Check sheet for the modelled part. Datum: model origin and axes. Units: mm. Face numbers are marked on the shaded views. A direction names the side the tool comes from. Round coordinates to 2 decimals unless told otherwise and drop trailing zeros. Write each loop counter-clockwise with the first axis right and the second up, starting at its lowest first coordinate (ties: lowest second). Pieces come first, ordered by that corner, then holes. Notation, with made-up numbers: M 73,-34 L 113,-34 A19 ccw 113,-1 Z; hole C 80.5,38 d1. An arc over 180 degrees is marked long. Answer in a Markdown table with one row per item.
```python
from build123d import *

# Parameters (mm, degrees)
SKETCH1_W           = 10
SKETCH1_H           = 80
BOSS_EXTRUDE1_DEPTH = 20
FILLET1_R           = 5
SKETCH3_R           = 3.99
BOSS_EXTRUDE2_DEPTH = 8.5
SKETCH4_R           = 5.65
BOSS_EXTRUDE3_DEPTH = 1.5
SKETCH2_R           = 5.65
BOSS_EXTRUDE4_DEPTH = 3
SKETCH6_R           = 3.99
BOSS_EXTRUDE5_DEPTH = 7.5
BOSS_EXTRUDE6_START = 3
SKETCH7_R           = 5.65
BOSS_EXTRUDE6_DEPTH = 3
BOSS_EXTRUDE7_START = 7.5
SKETCH9_R           = 3.99
BOSS_EXTRUDE7_DEPTH = 7.5


with BuildPart() as part:
    # Sketch1 → Boss-Extrude1 (new body)
    with BuildSketch(Plane(origin=(0, 0, 0), x_dir=(1, 0, 0), z_dir=(0, 1, 0))):
        with Locations((5, 40)):
            Rectangle(SKETCH1_W, SKETCH1_H)
    extrude(amount=BOSS_EXTRUDE1_DEPTH)

    # Fillet1
    fillet1_edges = [part.edges().sort_by_distance(p)[0] for p in [
        (5, 0, 0),
        (5, 20, 0),
    ]]
    fillet(fillet1_edges, radius=FILLET1_R)

    # Sketch3 → Boss-Extrude2 (add)
    with BuildSketch(Plane(origin=(0, 0, -80), x_dir=(-1, 0, 0), z_dir=(0, 0, -1))):
        with Locations(Location((-5, 10, 0), (0, 0, 180))):
            Circle(SKETCH3_R)
    extrude(amount=BOSS_EXTRUDE2_DEPTH)

    # Sketch4 → Boss-Extrude3 (add)
    with BuildSketch(Plane(origin=(0, 0, -80), x_dir=(-1, 0, 0), z_dir=(0, 0, -1))):
        with Locations(Location((-5, 10, 0), (0, 0, 207.753923356))):
            Circle(SKETCH4_R)
    extrude(amount=BOSS_EXTRUDE3_DEPTH)

    # Sketch2 → Boss-Extrude4 (add)
    with BuildSketch(Plane(origin=(10, 0, 0), x_dir=(0, 0, -1), z_dir=(1, 0, 0))):
        with Locations(Location((10, 10, 0), (0, 0, 180))):
            Circle(SKETCH2_R)
    extrude(amount=BOSS_EXTRUDE4_DEPTH)

    # Sketch6 → Boss-Extrude5 (add)
    with BuildSketch(Plane(origin=(13, 0, 0), x_dir=(0, 0, -1), z_dir=(1, 0, 0))):
        with Locations((10, 10)):
            Circle(SKETCH6_R)
    extrude(amount=BOSS_EXTRUDE5_DEPTH)

    # Sketch7 → Boss-Extrude6 (add)
    with BuildSketch(Plane.ZY.offset(BOSS_EXTRUDE6_START)):
        with Locations((-10, 10)):
            Circle(SKETCH7_R)
    extrude(amount=-BOSS_EXTRUDE6_DEPTH)

    # Sketch9 → Boss-Extrude7 (add)
    with BuildSketch(Plane.ZY.offset(3).offset(BOSS_EXTRUDE7_START)):
        with Locations(Location((-10, 10, 0), (0, 0, 180))):
            Circle(SKETCH9_R)
    extrude(amount=-BOSS_EXTRUDE7_DEPTH)


solid = part.part
```
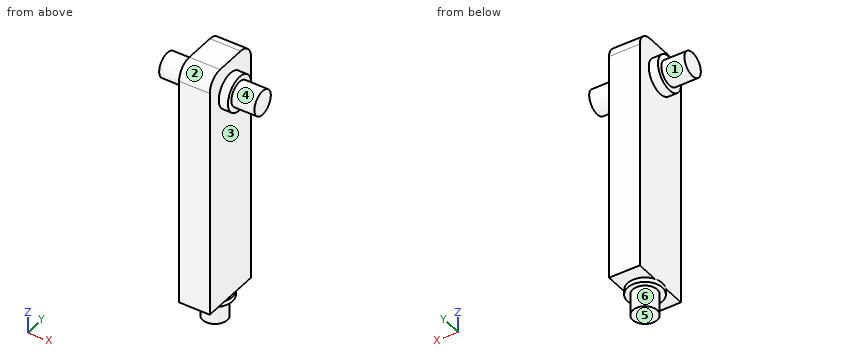
1. Access from +Z, -Z, +X, -X, +Y, -Y to the whole of each face (thin tool, end or side, straight path). Record for the marked faces 4, 5 and 6.
Found:
| item | result |
|---|---|
| face 4 | +X |
| face 5 | -Z, +X, -X, +Y, -Y |
| face 6 | -Z |
2. Section check A-A, the plane y = 10. Record the cut outline in (x, z).
Found:
| item | result |
|---|---|
| outline | M -10.5,-13.99 L -3,-13.99 L -3,-15.65 L 0,-15.65 L 0,-80 L -0.65,-80 L -0.65,-81.5 L 1.01,-81.5 L 1.01,-88.5 L 8.99,-88.5 L 8.99,-81.5 L 10.65,-81.5 L 10.65,-80 L 10,-80 L 10,-15.65 L 13,-15.65 L 13,-13.99 L 20.5,-13.99 L 20.5,-6.01 L 13,-6.01 L 13,-4.35 L 10,-4.35 L 10,0 L 0,0 L 0,-4.35 L -3,-4.35 L -3,-6.01 L -10.5,-6.01 Z |
3. Scan lines: L1, parallel to X at y = 10, z = -63.5; L2, parallel to Z at x = 8, y = 6; L3, parallel to Z at x = 8, y = 2.5. Record each from-to range of solid material in increasing order.
Found:
| item | result |
|---|---|
| L1 | x = 0 to 10 |
| L2 | z = -81.5 to 0 |
| L3 | z = -80 to -0.67 |
4. Section check C-C, the plane x = 18. Record the cut outline in (y, z).
Found:
| item | result |
|---|---|
| outline | C 10,-10 d7.98 |
5. Go/stop test with flat-tipped pins: pin 1 (1.5 mm diameter, centred on y = 9.5, z = -79, fed in from +X); pin 2 (2 mm diameter, centred on x = -7.5, y = 12, fed in from +Z); pin 3 (4 mm diameter, centred on x = 4.5, y = 2, fed in from +Z). Record where each tip stops, or that it passes through.
Found:
| item | result |
|---|---|
| pin 1 | stops at x = 10 |
| pin 2 | stops at z = -6.14 |
| pin 3 | stops at z = -0.1 |
6. Draft check along Z on the marked faces 1, 2 and 3. Enter one of: +Z half, -Z half, draft (parallel to the pull), parting line (faces both ways), or undercut.
Found:
| item | result |
|---|---|
| face 1 | parting line |
| face 2 | +Z half |
| face 3 | undercut |
7. Section check D-D, the plane z = -27.5. Record the cut outline in (x, y), and give its area (3 significant figures).
Found:
| item | result |
|---|---|
| outline | M 0,0 L 10,0 L 10,20 L 0,20 Z |
| area | 200 mm2 |
8. Section check B-B, the plane z = -10. Record the cut outline in (x, y), and give its area (4 significant figures).
Found:
| item | result |
|---|---|
| outline | M -10.5,6.01 L -3,6.01 L -3,4.35 L 0,4.35 L 0,0 L 10,0 L 10,4.35 L 13,4.35 L 13,6.01 L 20.5,6.01 L 20.5,13.99 L 13,13.99 L 13,15.65 L 10,15.65 L 10,20 L 0,20 L 0,15.65 L -3,15.65 L -3,13.99 L -10.5,13.99 Z |
| area | 387.5 mm2 |
